from build123d import *

# Parameters (mm, degrees)
SKETCH1_R           = 37.5
BOSS_EXTRUDE1_DEPTH = 15
SKETCH2_R           = 21.1
CUT_EXTRUDE1_DEPTH  = 7.8
SKETCH3_R           = 17
CUT_EXTRUDE2_DEPTH  = 8.2
SKETCH4_R           = 2.1
CUT_EXTRUDE3_DEPTH  = 16
CHAMFER1_SIZE       = 7
CHAMFER1_SIZE2      = 8.342275148


with BuildPart() as part:
    # Sketch1 → Boss-Extrude1 (new body)
    with BuildSketch(Plane(origin=(0, 0, 0), x_dir=(1, 0, 0), z_dir=(0, 1, 0))):
        with Locations(Location((0, 0, 0), (0, 0, 270))):  # turned: the seam where the file's is
            Circle(SKETCH1_R)
    extrude(amount=BOSS_EXTRUDE1_DEPTH)

    # Sketch2 → Cut-Extrude1 (cut)
    with BuildSketch(Plane.XZ):
        with Locations(Location((0, 0, 0), (0, 0, 270))):  # turned: the seam where the file's is
            Circle(SKETCH2_R)
    extrude(amount=-CUT_EXTRUDE1_DEPTH, mode=Mode.SUBTRACT)

    # Sketch3 → Cut-Extrude2 (cut, through all)
    with BuildSketch(Plane.XZ.offset(-7.8)):
        with Locations(Location((0, 0, 0), (0, 0, 270))):  # turned: the seam where the file's is
            Circle(SKETCH3_R)
    extrude(amount=-CUT_EXTRUDE2_DEPTH, mode=Mode.SUBTRACT)

    # Sketch4 → Cut-Extrude3 (cut, through all)
    with BuildSketch(Plane(origin=(0, 15, 0), x_dir=(1, 0, 0), z_dir=(0, 1, 0))):
        with Locations(Location((-21, -21, 0), (0, 0, 270))):  # turned: the seam where the file's is
            Circle(SKETCH4_R)
        with Locations(Location((-21, 21, 0), (0, 0, 270))):  # turned: the seam where the file's is
            Circle(SKETCH4_R)
        with Locations(Location((21, 21, 0), (0, 0, 270))):  # turned: the seam where the file's is
            Circle(SKETCH4_R)
        with Locations(Location((21, -21, 0), (0, 0, 270))):  # turned: the seam where the file's is
            Circle(SKETCH4_R)
    extrude(amount=-CUT_EXTRUDE3_DEPTH, mode=Mode.SUBTRACT)

    # Chamfer1
    chamfer1_edges = [part.edges().sort_by_distance(p)[0] for p in [
        (0, 15, 17),
    ]]
    chamfer1_side = [part.faces().sort_by_distance(p)[0] for p in [
        (0, 11.4, 17),
    ]]
    chamfer(chamfer1_edges, length=CHAMFER1_SIZE, length2=CHAMFER1_SIZE2, reference=chamfer1_side[0])


solid = part.part
Read the model definition and answer for the solid it produces. Units are mm, in the model's axes. A direction names the side the tool comes from. Give positions to 0.01 mm unless a question says otherwise; leave off trailing zeros. Write each loop counter-clockwise with the first axis right and the second up, starting at its lowest first coordinate (ties: lowest second). Pieces come first, ordered by that corner, then holes. Notation, with made-up numbers: (46.5, -15.75) - (55.5, -15.75) arc R6 cw to (55.5, -4.75) - close; hole circle Ø4 at (-36.5, 38). An arc over 180 degrees is marked (long way). Use CSV: the item, a comma, the result in double quotes. Start each with the question number.
(1) Find section B-B (x = 0). Give the vertices of the cut face in (y, z), plus the area to 3 significant figures.
(2) Find section C-C (y = 4). Give the vertices of the cut face in (x, z).
(3) Consider line 1 along X through (y, z) = (6.25, 0); line 2 along X through (y, z) = (10, -21); line 3 along X through (y, z) = (2, -6.5). Determine where each line is inside the solid, lowest interval first.
(4) Determine the mould class of faces 3 (the cylindrical face through (21.631, 7.605, 23.003)), 4 (the cylindrical face through (-19.23, 7.6, 22.13)), 5 (the cylindrical face through (-22.818, 7.395, -29.759)), 6 (the flat face through (-24.5, 15, 7.8)) for opening direction Z: +Z half, -Z half, draft (parallel to the pull), parting line (faces both ways), or undercut.
(5) Find section A-A (z = 0). Give the vertices of the cut face in (x, y), plus the area to 3 significant figures.
(6) Find section D-D (z = -28). Give the vertices of the cut face in (x, y).
(7) For faces 1 (the flat face through (17.3, 7.8, -1.5)), 2 (the conical face through (5.263, 8.438, -16.713)), determine the directions among +Z, -Z, +X, -X, +Y, -Y from which every point of the face is accessible in a straight line to the end or side of a thin tool.
(8) Given P1, Ø5, axis at y = 2.5, z = 28.5, coming from the -X side; P2, Ø1.5, axis at y = 10.5, z = -4, coming from the +X side; P3, Ø8, axis at y = 6.5, z = 10, coming from the +X side, each flat-ended and moving along its own axis, determine where each tip first touches the part or whether it passes through.
Findings below:
1,outline,"(0, -37.5) - (15, -37.5) - (15, -25.34) - (8, -17) - (7.8, -17) - (7.8, -21.1) - (0, -21.1) - close; (0, 21.1) - (7.8, 21.1) - (7.8, 17) - (8, 17) - (15, 25.34) - (15, 37.5) - (0, 37.5) - close"
1,area,"493 mm2"
2,outline,"circle Ø75 at (0, 0); hole circle Ø4.2 at (-21, -21); hole circle Ø4.2 at (-21, 21); hole circle Ø42.2 at (0, 0); hole circle Ø4.2 at (21, -21); hole circle Ø4.2 at (21, 21)"
3,line 1,"-37.5 to -21.1, 21.1 to 37.5"
3,line 2,"-31.07 to -23.1, -18.9 to 18.9, 23.1 to 31.07"
3,line 3,"-36.93 to -20.07, 20.07 to 36.93"
4,face 3,"undercut"
4,face 4,"undercut"
4,face 5,"parting line"
4,face 6,"draft"
5,outline,"(-37.5, 0) - (-21.1, 0) - (-21.1, 7.8) - (-17, 7.8) - (-17, 8) - (-25.34, 15) - (-37.5, 15) - close; (17, 7.8) - (21.1, 7.8) - (21.1, 0) - (37.5, 0) - (37.5, 15) - (25.34, 15) - (17, 8) - close"
5,area,"493 mm2"
6,outline,"(-24.94, 0) - (24.94, 0) - (24.94, 15) - (-24.94, 15) - close"
7,face 1,"-Y"
7,face 2,"+Y"
8,P1,"x = -27.02"
8,P2,"x = 37.36"
8,P3,"x = 37.02"
